The listing builds one solid part. Answer for the finished solid, in the listing's coordinates (mm). A direction names the side the tool comes from. Coordinates: 2 decimals unless noted, no trailing zeros. Order: outer loops, then holes, each group sorted by start corner. A loop starts at its lowest first (then second) coordinate and runs counter-clockwise, first axis right, second up.
```python
from build123d import *

# Parameters (mm, degrees)
F1_DEPTH = 990.6
F2_R     = 6.35
F3_DEPTH = 25.4


with BuildPart() as f1:
    # F0 (on Front) → F1 (new body)
    with BuildSketch(Plane.XZ):
        Polygon((-6.35, 0), (0, 0), (0, 38.1), (-63.5, 38.1), (-63.5, 31.75), (-6.35, 31.75), align=None)
    extrude(amount=F1_DEPTH)

    # F2 (on face) → F3 (cut)
    with BuildSketch(Plane.XY.offset(38.1)):
        with Locations((-47.625, -952.5)):
            Circle(F2_R)
        with Locations((-47.625, -647.7)):
            Circle(F2_R)
        with Locations((-47.625, -342.9)):
            Circle(F2_R)
        with Locations((-47.625, -38.1)):
            Circle(F2_R)
    extrude(amount=-F3_DEPTH, mode=Mode.SUBTRACT)


solid = f1.part
```
1) The mould has two halves that part along X. Classify faces 3 (the flat face through (-31, -488, 38.1)), 4 (the flat face through (0, -488, 19)), 5 (the flat face through (-6.35, -488, 16)): released by +X, released by -X, zero draft, split by the parting line, or undercut.
2) Straight lines are drawn through the part: probe 1 along X at (y, z) = (-952.5, 34.75) (3 decimals); probe 2 along Z at (x, y) = (-47.5, -561.5); probe 3 along X at (y, z) = (-516.5, 26). For each, find the intervals that lie inside material, in ascending order.
3) A cutting plane is placed at A-A, the plane y = -929. Write down the section's boundary in (x, z).
4) A cutting plane is placed at B-B, the plane x = -22. Write down the section's boundary in (y, z).
5) Each of these flat-tipped pins is pushed along its axis until it touches: P1, Ø3, axis at y = -703, z = 7, coming from the -X side; P2, Ø16.5, axis at x = -47.625, y = -952.5, coming from the -Z side; P3, Ø11.5, axis at x = -47.625, y = -342.9, coming from the +Z side. Where does it stop, or does it pass through?
6) For faces 1 (the flat face through (-22, 0, 32)), 2 (the flat face through (-35, -488, 31.75)), determine the directions among +Z, -Z, +X, -X, +Y, -Y from which every point of the face is accessible in a straight line to the end or side of a thin tool.
Working result:
1. face 3: zero draft
1. face 4: released by +X
1. face 5: released by -X
2. probe 1: x = -63.5 to -53.975, -41.275 to 0
2. probe 2: z = 31.75 to 38.1
2. probe 3: x = -6.35 to 0
3. outline: (-63.5, 31.75) - (-6.35, 31.75) - (-6.35, 0) - (0, 0) - (0, 38.1) - (-63.5, 38.1) - close
4. outline: (-990.6, 31.75) - (0, 31.75) - (0, 38.1) - (-990.6, 38.1) - close
5. P1: stops at x = -6.35
5. P2: stops at z = 31.75
5. P3: passes through
6. face 1: +Z, -Z, +X, -X, +Y
6. face 2: -Z, -X, +Y, -Y
